Check sheet for the modelled part. Datum: model origin and axes. Units: mm. Round coordinates to 2 decimals unless told otherwise and drop trailing zeros. Order: outer loops, then holes, each group sorted by start corner. A loop starts at its lowest first (then second) coordinate and runs counter-clockwise, first axis right, second up.
```python
from build123d import *

# Parameters (mm, degrees)
BOSS_EXTRUDE1_DEPTH     = 3
SKETCH9_W               = 14
SKETCH9_H               = 4
CUT_EXTRUDE3_DEPTH      = 4.0000001
CUT_EXTRUDE4_DEPTH      = 1.0000001
CUT_EXTRUDE4_DEPTH_BACK = 3


with BuildPart() as part:
    # Sketch1 → Boss-Extrude1 (new body)
    with BuildSketch(Plane.XY):
        with BuildLine():
            Line((-39, 0), (-8, 0))
            Line((-8, 0), (-7.5, 7.002171092))
            Line((-7.5, 7.002171092), (-7, 7.002171092))
            Line((-7, 7.002171092), (-7, -1.997828908))
            Line((-7, -1.997828908), (-7.5, -2.997828908))
            Line((-7.5, -2.997828908), (-8, -3.497828908))
            Line((-8, -3.497828908), (-8, -4.497828908))
            Line((-8, -4.497828908), (-6.5, -5.997828908))
            Line((-6.5, -5.997828908), (-5, -5.997828908))
            Line((-5, -5.997828908), (-4.5, 7.002171092))
            Line((-4.5, 7.002171092), (-4, 7.002171092))
            Line((-4, 7.002171092), (-4, -5.997828908))
            Line((-4, -5.997828908), (4, -5.997828908))
            Line((4, -5.997828908), (4, 7.002171092))
            Line((4, 7.002171092), (4.5, 7.002171092))
            Line((4.5, 7.002171092), (5, -5.997828908))
            Line((5, -5.997828908), (6.5, -5.997828908))
            Line((6.5, -5.997828908), (8, -4.497828908))
            Line((8, -4.497828908), (8, -3.497828908))
            Line((8, -3.497828908), (7.5, -2.997828908))
            Line((7.5, -2.997828908), (7, -1.997828908))
            Line((7, -1.997828908), (7, 7.002171092))
            Line((7, 7.002171092), (7.5, 7.002171092))
            Line((7.5, 7.002171092), (8, 0))
            Line((8, 0), (38.94, 0))
            add(Edge.make_bspline(
                [(38.94, 0), (38.94, 30.292119235), (27.145, 56)],
                knots=[1.570796327, 1.570796327, 1.570796327, 2.128135243, 2.128135243, 2.128135243], degree=2, weights=[1, 0.96142229, 1]))
            Line((27.145, 56), (14, 56))
            Line((14, 56), (13.5, 48.997828908))
            Line((13.5, 48.997828908), (13, 48.997828908))
            Line((13, 48.997828908), (13, 57.997828908))
            Line((13, 57.997828908), (13.5, 58.997828908))
            Line((13.5, 58.997828908), (14, 59.497828908))
            Line((14, 59.497828908), (14, 60.497828908))
            Line((14, 60.497828908), (12.5, 61.997828908))
            Line((12.5, 61.997828908), (11, 61.997828908))
            Line((11, 61.997828908), (10.5, 48.997828908))
            Line((10.5, 48.997828908), (10, 48.997828908))
            Line((10, 48.997828908), (10, 61.997828908))
            Line((10, 61.997828908), (2, 61.997828908))
            Line((2, 61.997828908), (2, 48.997828908))
            Line((2, 48.997828908), (1.5, 48.997828908))
            Line((1.5, 48.997828908), (1, 61.997828908))
            Line((1, 61.997828908), (-0.5, 61.997828908))
            Line((-0.5, 61.997828908), (-2, 60.497828908))
            Line((-2, 60.497828908), (-2, 59.497828908))
            Line((-2, 59.497828908), (-1.5, 58.997828908))
            Line((-1.5, 58.997828908), (-1, 57.997828908))
            Line((-1, 57.997828908), (-1, 48.997828908))
            Line((-1, 48.997828908), (-1.5, 48.997828908))
            Line((-1.5, 48.997828908), (-2, 56))
            Line((-2, 56), (-46, 56))
            Line((-46, 56), (-46.5, 48.997828908))
            Line((-46.5, 48.997828908), (-47, 48.997828908))
            Line((-47, 48.997828908), (-47, 57.997828908))
            Line((-47, 57.997828908), (-46.5, 58.997828908))
            Line((-46.5, 58.997828908), (-46, 59.497828908))
            Line((-46, 59.497828908), (-46, 60.497828908))
            Line((-46, 60.497828908), (-47.5, 61.997828908))
            Line((-47.5, 61.997828908), (-49, 61.997828908))
            Line((-49, 61.997828908), (-49.5, 48.997828908))
            Line((-49.5, 48.997828908), (-50, 48.997828908))
            Line((-50, 48.997828908), (-50, 61.997828908))
            Line((-50, 61.997828908), (-58, 61.997828908))
            Line((-58, 61.997828908), (-58, 48.997828908))
            Line((-58, 48.997828908), (-58.5, 48.997828908))
            Line((-58.5, 48.997828908), (-59, 61.997828908))
            Line((-59, 61.997828908), (-60.5, 61.997828908))
            Line((-60.5, 61.997828908), (-62, 60.497828908))
            Line((-62, 60.497828908), (-62, 59.497828908))
            Line((-62, 59.497828908), (-61.5, 58.997828908))
            Line((-61.5, 58.997828908), (-61, 57.997828908))
            Line((-61, 57.997828908), (-61, 48.997828908))
            Line((-61, 48.997828908), (-61.5, 48.997828908))
            Line((-61.5, 48.997828908), (-62, 56))
            Line((-62, 56), (-105.145, 56))
            add(Edge.make_bspline(
                [(-105.145, 56), (-116.94, 30.292119235), (-116.94, 0)],
                knots=[4.155050064, 4.155050064, 4.155050064, 4.71238898, 4.71238898, 4.71238898], degree=2, weights=[1, 0.96142229, 1]))
            Line((-116.94, 0), (-86, 0))
            Line((-86, 0), (-85.5, 7.002171092))
            Line((-85.5, 7.002171092), (-85, 7.002171092))
            Line((-85, 7.002171092), (-85, -1.997828908))
            Line((-85, -1.997828908), (-85.5, -2.997828908))
            Line((-85.5, -2.997828908), (-86, -3.497828908))
            Line((-86, -3.497828908), (-86, -4.497828908))
            Line((-86, -4.497828908), (-84.5, -5.997828908))
            Line((-84.5, -5.997828908), (-83, -5.997828908))
            Line((-83, -5.997828908), (-82.5, 7.002171092))
            Line((-82.5, 7.002171092), (-82, 7.002171092))
            Line((-82, 7.002171092), (-82, -5.997828908))
            Line((-82, -5.997828908), (-74, -5.997828908))
            Line((-74, -5.997828908), (-74, 7.002171092))
            Line((-74, 7.002171092), (-73.5, 7.002171092))
            Line((-73.5, 7.002171092), (-73, -5.997828908))
            Line((-73, -5.997828908), (-71.5, -5.997828908))
            Line((-71.5, -5.997828908), (-70, -4.497828908))
            Line((-70, -4.497828908), (-70, -3.497828908))
            Line((-70, -3.497828908), (-70.5, -2.997828908))
            Line((-70.5, -2.997828908), (-71, -1.997828908))
            Line((-71, -1.997828908), (-71, 7.002171092))
            Line((-71, 7.002171092), (-70.5, 7.002171092))
            Line((-70.5, 7.002171092), (-70, 0))
            Line((-70, 0), (-39, 0))
        make_face()
    extrude(amount=BOSS_EXTRUDE1_DEPTH)

    # Sketch9 → Cut-Extrude3 (cut, through all)
    with BuildSketch(Plane.XY.offset(3)):
        with Locations((-24, 54)):
            Rectangle(SKETCH9_W, SKETCH9_H)
        with Locations((-84, 54)):
            Rectangle(SKETCH9_W, SKETCH9_H)
    extrude(amount=-CUT_EXTRUDE3_DEPTH, mode=Mode.SUBTRACT)

    # Sketch11 → Cut-Extrude4 (cut, two sides)
    with BuildSketch(Plane.XY.offset(3)) as cut_extrude4_sk:
        Polygon((-40.5, 267.538526516), (-40.5, 56), (-40.5, 28), (-37.5, 28), (-37.5, 56), (-37.5, 267.538526516), (-37.5, 690.615579549), (-40.5, 690.615579549), align=None)
    extrude(amount=CUT_EXTRUDE4_DEPTH, mode=Mode.SUBTRACT)
    extrude(cut_extrude4_sk.sketch, amount=-CUT_EXTRUDE4_DEPTH_BACK, mode=Mode.SUBTRACT)


solid = part.part
```
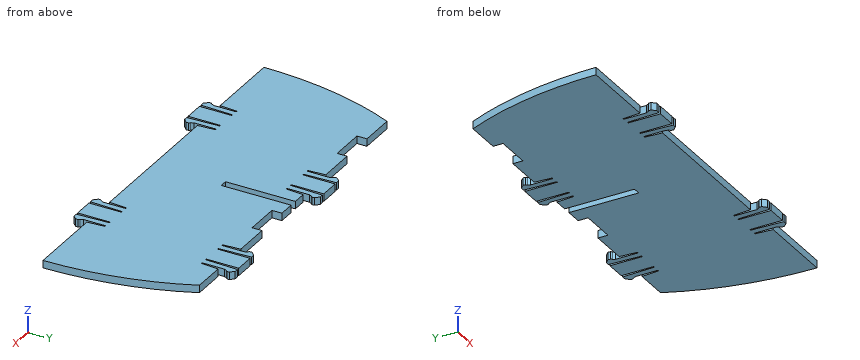
Item 1: Sectioned sample at B-B (y = 54). State how many separate pieces and enclosed holes the cut face has, and give its area (3 significant figures).
Answer:
separate pieces: 12
enclosed holes: 0
area: 291 mm2
Item 2: Sectioned sample at A-A (x = -35). Record the cut outline in (y, z).
Answer:
outline: (0, 0) - (56, 0) - (56, 3) - (0, 3) - close
Item 3: Scan lines: line 1 along Y through (x, z) = (-36, 2.5); line 2 along X through (y, z) = (40.5, 0.5); line 3 along X through (y, z) = (46.5, 2.1). Record each from-to range of solid material in increasing order.
Answer:
line 1: y = 0 to 56
line 2: x = -111.01 to -40.5, -37.5 to 33.01
line 3: x = -109.02 to -40.5, -37.5 to 31.02
Item 4: Go/stop test with flat-tipped pins: P1, Ø0.5, axis at y = 60, z = 2, coming from the -X side; P2, Ø1.5, axis at y = 55, z = 1.5, coming from the +X side; P3, Ø1, axis at y = 28.5, z = 2.5, coming from the -X side (3 decimals); P4, Ø4, axis at x = -29, y = 39.5, coming from the -Z side. Record where each tip stops, or that it passes through.
Answer:
P1: stops at x = -62
P2: stops at x = 27.93
P3: stops at x = -114.165
P4: stops at z = 0
